Here's how the part is built. I have some questions about the finished solid (model axes, mm). A direction names the side the tool comes from. Give positions to 0.01 mm unless a question says otherwise; leave off trailing zeros. Loops run counter-clockwise (first coordinate to the right, second up) from the corner with the lowest first, then second, coordinate; pieces in that order, holes last. Notation, with made-up numbers: (-15, -25) -> (36, -25) arc R12 ccw to (36, -20) -> close; hole circle Ø7 at (44, 5). An arc over 180 degrees is marked (long way). Answer in a Markdown table with one row per item. Add a question column.
Item 1: We'd pull the mould along X, two halves only. Please class faces 3 (the face through (-104, 3, -241.3)), 4 (the face through (-104, 3, -21.431)), 5 (the face through (-202.616, 3.131, -118.961)): released by +X, released by -X, zero draft, split by the parting line, or undercut.
Item 2: Which directions (+Z, -Z, +X, -X, +Y, -Y) give clear straight access to the entire face, cutting with the end or side of a thin tool? Please do faces 1 (the face through (-102, 3, -219.869)), 2 (the face through (-192, 6.35, -119)).
Item 3: For P1, Ø2, axis at y = 2.5, z = -56.5, coming from the -X side; P2, Ø1.5, axis at y = 4, z = -51.5, coming from the -X side; P3, Ø12, axis at x = -62, z = -209.5, coming from the +Y side, each with a flat end and sliding along its axis, tell me the tip position at first contact or that it passes through.
Item 4: If we section it at C-C (y = 4): Write out the boundary of the cut face in (x, z) (3 decimals), then the cut area to 3 significant figures.
Item 5: If I drill on line 1 (Z direction, x = -157.5, y = 2.25); line 2 (X direction, y = 3.5, z = -216) (3 decimals); line 3 (X direction, y = 2.5, z = -42.5) (3 decimals), over which ranges is the centre line in solid material (lowest first)?
Item 6: If we section it at A-A (x = -175): Write out the boundary of the cut face in (y, z), then the cut area to 3 significant figures.
Autodesk Inventor part; units mm, degrees
ref_plane "YZ Plane" through (0, 0, 0) normal (1, 0, 0) x (0, 1, 0)
ref_plane "XZ Plane" through (0, 0, 0) normal (0, 1, 0) x (-1, 0, 0)
ref_plane "XY Plane" through (0, 0, 0) normal (0, 0, 1) x (1, 0, 0)
sketch "Sketch1" plane through (0, 0, 0) normal (0, 1, 0) x (-1, 0, 0)
  line L0 (0, 0) -> (204.7875, 0)
  line L1 (204.7875, 0) -> (204.7875, -241.3)
  line L2 (204.7875, -241.3) -> (0, -241.3)
  line L3 (0, -241.3) -> (0, 0)
  dimension "d0" = 204.7875
  dimension "d1" = 241.3
extrude "Extrusion1" add sketch "Sketch1" along normal blind 6.35
sketch "Sketch2" plane through (0, 6.35, 0) normal (0, 1, 0) x (1, 0, 0)
  line L0 (-28.575, 219.8688) -> (-177.8, 219.8688)
  line L1 (-177.8, 219.8688) -> (-177.8, 21.4312)
  line L2 (-177.8, 21.4312) -> (-28.575, 21.4313)
  line L3 (-28.575, 21.4313) -> (-28.575, 219.8688)
  line L4 (0, 0) -> (-204.7875, 0)
  line L5 (-204.7875, 241.3) -> (-204.7875, 0)
  dimension "d4" = 149.225
  dimension "d5" = 198.4375
  dimension "d6" = 21.4312
  dimension "d7" = 26.9875
extrude "Extrusion2" cut sketch "Sketch2" against normal blind 25.4
sketch "Sketch4" plane through (-204.7875, 0, 0) normal (0, 0, 1) x (1, 0, 0)
  line L0 (4.2831, 0) -> (-0.0504, 6.4246)
  line L1 (0, 0) -> (0, 6.35)
  line L2 (204.7875, 0) -> (0, 0)
  line L3 (0, 6.35) -> (0, 0)
  line L4 (0, 0) -> (4.2831, 0)
extrude "Extrusion4" cut sketch "Sketch4" against normal blind 241.3
properties part number "screen_holder"
Recorded:
| question | item | result |
|---|---|---|
| 1 | face 3 | zero draft |
| 1 | face 4 | undercut |
| 1 | face 5 | released by -X |
| 2 | face 1 | +Y, -Y |
| 2 | face 2 | +Z, -Z, +X, -X, +Y |
| 3 | P1 | stops at x = -202.87 |
| 3 | P2 | stops at x = -203.71 |
| 3 | P3 | passes through |
| 4 | outline | (-203.202, -241.3) -> (0, -241.3) -> (0, 0) -> (-203.202, 0) -> close; hole (-177.8, -219.869) -> (-28.575, -219.869) -> (-28.575, -21.431) -> (-177.8, -21.431) -> close |
| 4 | area | 19,400 mm^2 |
| 5 | line 1 | z = -241.3 to -219.87, -21.43 to 0 |
| 5 | line 2 | x = -202.865 to -177.8, -28.575 to 0 |
| 5 | line 3 | x = -202.191 to -177.8, -28.575 to 0 |
| 6 | outline | (0, -241.3) -> (6.35, -241.3) -> (6.35, -219.87) -> (0, -219.87) -> close; (0, -21.43) -> (6.35, -21.43) -> (6.35, 0) -> (0, 0) -> close |
| 6 | area | 272 mm^2 |
